from build123d import *

# Parameters (mm, degrees)
BOSS_EXTRUDE1_DEPTH = 50
SKETCH2_W           = 20
SKETCH2_H           = 30
CUT_EXTRUDE1_DEPTH  = 50
SKETCH3_R           = 7.5
CUT_EXTRUDE2_DEPTH  = 50
SKETCH4_W           = 10
SKETCH4_H           = 10
BOSS_EXTRUDE2_DEPTH = 40
EXTRUDE_THIN1_DEPTH = 10
BOSS_EXTRUDE3_DEPTH = 10


with BuildPart() as part:
    # Sketch1 → Boss-Extrude1 (new body)
    with BuildSketch(Plane.XY):
        Polygon((-7.5, 25), (-7.5, -10), (47.5, -10), (47.5, -25), (-47.5, -25), (-47.5, 25), align=None)
    extrude(amount=-BOSS_EXTRUDE1_DEPTH)

    # Sketch2 → Cut-Extrude1 (cut)
    with BuildSketch(Plane(origin=(0, 25, 0), x_dir=(1, 0, 0), z_dir=(0, 1, 0))):
        with Locations((-27.5, 25)):
            Rectangle(SKETCH2_W, SKETCH2_H)
    extrude(amount=-CUT_EXTRUDE1_DEPTH, mode=Mode.SUBTRACT)

    # Sketch3 → Cut-Extrude2 (cut)
    with BuildSketch(Plane.XY):
        with Locations((-27.5, 0)):
            Circle(SKETCH3_R)
    extrude(amount=-CUT_EXTRUDE2_DEPTH, mode=Mode.SUBTRACT)

    # Sketch4 → Boss-Extrude2 (add)
    with BuildSketch(Plane(origin=(0, 25, 0), x_dir=(1, 0, 0), z_dir=(0, 1, 0))):
        with Locations((-2.5, 25)):
            Rectangle(SKETCH4_W, SKETCH4_H)
    extrude(amount=-BOSS_EXTRUDE2_DEPTH)

    # Sketch7 → Extrude-Thin1 (add)
    with BuildSketch(Plane.XY.offset(-20)):
        Polygon((2.5, 25), (47.5, -10), (41.360593865, -17.893522174), (-3.639406135, 17.106477826), align=None)
    extrude(amount=-EXTRUDE_THIN1_DEPTH)

    # Sketch8 → Boss-Extrude3 (add)
    with BuildSketch(Plane.XY.offset(-20)):
        Polygon((2.5, -10), (2.5, 12.331384166), (31.211779641, -10), align=None)
    extrude(amount=-BOSS_EXTRUDE3_DEPTH)


solid = part.part
Could you check a few things on this model? Use its own coordinates, in mm. A direction names the side the tool comes from. Coordinates: 2 decimals unless noted, no trailing zeros. Order: outer loops, then holes, each group sorted by start corner. A loop starts at its lowest first (then second) coordinate and runs counter-clockwise, first axis right, second up.
Q1. Suppose I cut it at B-B on z = -18. Please give me the cut outline in (x, y).
Q2. Which directions (+Z, -Z, +X, -X, +Y, -Y) give clear straight access to the entire face, cutting with the end or side of a thin tool? Please do faces 5 (the flat face through (20, -10, -40)), 6 (the cylindrical face through (-35, 0, -5)), 7 (the flat face through (-34, 6, -10)), 8 (the flat face through (24.685, 7.745, -24.93)), 9 (the flat face through (-7.5, 8, -10)).
Q3. Thinking about a two-plate mould opening in Z: for faces 1 (the cylindrical face through (-35, 0, -45)), 2 (the flat face through (-10, -5, -50)), 3 (the flat face through (-37.5, 0, -25)), 4 (the flat face through (14, 4, -20)), which applies, released by +Z, released by -Z, zero draft, split by the parting line, or undercut?
Q4. Will these pins go through, and if not, where does the flat tip stop? pin 1 (22 mm diameter, centred on y = 3, z = -11.5, fed in from +X); pin 2 (2 mm diameter, centred on x = -2, y = 10, fed in from -Z); pin 3 (10 mm diameter, centred on x = 27.5, z = -19, fed in from +Y); pin 4 (24 mm diameter, centred on x = -27.5, y = 0, fed in from +Z).
Q5. Suppose I cut it at A-A on x = -27.5. Please give me the cut outline in (y, z).
Q6. Suppose I cut it at D-D on y = 0. Please give me the cut outline in (x, z).
Q7. Please list where these lines run through material, in increasing order: L1, parallel to Y at x = -27.5, z = -7.75; L2, parallel to X at y = -16.5, z = -10.5; L3, parallel to Z at x = -19, y = -22.5.
Q8. Suppose I cut it at C-C on y = -19. Please give me the cut outline in (x, z).
Answer:
1. outline: (-47.5, -25) - (-37.5, -25) - (-37.5, 25) - (-47.5, 25) - close; (-17.5, -25) - (47.5, -25) - (47.5, -10) - (-7.5, -10) - (-7.5, 25) - (-17.5, 25) - close
2. face 5: -Z, +X, +Y
2. face 6: +Z, -Z
2. face 7: +Y, -Y
2. face 8: +Z, -Z, +X, +Y
2. face 9: +Z, +X, +Y
3. face 1: zero draft
3. face 2: released by -Z
3. face 3: undercut
3. face 4: released by +Z
4. pin 1: stops at x = 39.76
4. pin 2: stops at z = -30
4. pin 3: stops at y = 9.37
4. pin 4: stops at z = 0
5. outline: (-25, -50) - (-7.5, -50) - (-7.5, -40) - (-25, -40) - close; (-25, -10) - (-7.5, -10) - (-7.5, 0) - (-25, 0) - close; (7.5, -50) - (25, -50) - (25, -40) - (7.5, -40) - close; (7.5, -10) - (25, -10) - (25, 0) - (7.5, 0) - close
6. outline: (-47.5, -50) - (-35, -50) - (-35, -40) - (-37.5, -40) - (-37.5, -10) - (-35, -10) - (-35, 0) - (-47.5, 0) - close; (-20, -50) - (-7.5, -50) - (-7.5, -30) - (34.64, -30) - (34.64, -20) - (-7.5, -20) - (-7.5, 0) - (-20, 0) - (-20, -10) - (-17.5, -10) - (-17.5, -40) - (-20, -40) - close
7. L1: y = -25 to -7.5, 7.5 to 25
7. L2: x = -47.5 to -37.5, -17.5 to 47.5
7. L3: z = -50 to -40, -10 to 0
8. outline: (-47.5, -50) - (47.5, -50) - (47.5, 0) - (-47.5, 0) - close; hole (-37.5, -40) - (-17.5, -40) - (-17.5, -10) - (-37.5, -10) - close
